```python
from build123d import *

# Parameters (mm, degrees)
F1_DEPTH = 38.1
F2_R     = 88.9
F3_DEPTH = 25.4
F5_DEPTH = 38.1


with BuildPart() as f1:
    # F0 (on Front) → F1 (new body)
    with BuildSketch(Plane.XZ):
        with BuildLine():
            Line((88.9, 0), (0, 0))
            Line((0, 0), (0, -127))
            ThreePointArc((0, -127), (7.4394877579, -144.9605122421), (25.4, -152.4))
            Line((25.4, -152.4), (63.5, -152.4))
            ThreePointArc((63.5, -152.4), (81.4605122421, -144.9605122421), (88.9, -127))
            Line((88.9, -127), (88.9, 0))
        make_face()
    extrude(amount=F1_DEPTH)

    # F2 (on face) → F3 (join)
    with BuildSketch(Plane.XZ.offset(38.1)):
        with Locations((44.45, -114.3)):
            Circle(F2_R)
    extrude(amount=F3_DEPTH)

    # F4 (on face) → F5 (join)
    with BuildSketch(Plane.XZ.offset(63.5)):
        with BuildLine():
            Line((88.9, 0), (0, 0))
            Line((0, 0), (0, -127))
            ThreePointArc((0, -127), (7.4394877579, -144.9605122421), (25.4, -152.4))
            Line((25.4, -152.4), (63.5, -152.4))
            ThreePointArc((63.5, -152.4), (81.4605122421, -144.9605122421), (88.9, -127))
            Line((88.9, -127), (88.9, 0))
        make_face()
    extrude(amount=F5_DEPTH)


solid = f1.part
```
Geometry check sheet. Reference: the model listing, model coordinates, mm. A direction names the side the tool comes from. Coordinates: 2 decimals unless noted, no trailing zeros. Write each loop counter-clockwise with the first axis right and the second up, starting at its lowest first coordinate (ties: lowest second). Pieces come first, ordered by that corner, then holes. Notation, with made-up numbers: M 50,88 L 106,88 A17 cw 106,108 Z; hole C -4.5,75.25 d2. An arc over 180 degrees is marked long. Answer as a JSON object with one key per item and string values.
1. Go/stop test with flat-tipped pins: pin 1 Ø18.5 at (x, z) = (41.5, -10.5) entering from +Y; pin 2 Ø4 at (x, y) = (78, -82.5) entering from -Z; pin 3 Ø12 at (y, z) = (-19, -155) entering from -X; pin 4 Ø12 at (y, z) = (-28.5, -91) entering from +X. Record where each tip stops, or that it passes through.
Answers below:
{"pin 1": "stops at y = 0", "pin 2": "stops at z = -149.11", "pin 3": "stops at x = 12.71", "pin 4": "stops at x = 88.9"}
2. Section check C-C, the plane y = -78. Enter the section's corners in (x, z), plus the area to 3 significant figures.
Answers below:
{"outline": "M 0,-127 A25.4 ccw 25.4,-152.4 L 63.5,-152.4 A25.4 ccw 88.9,-127 L 88.9,0 L 0,0 Z", "area": "13,300 mm²"}
3. Section check D-D, the plane y = -54.5. Enter the section's corners in (x, z).
Answers below:
{"outline": "C 44.45,-114.3 d177.8"}
4. Scan lines: L1, parallel to Y at x = -18.5, z = -94; L2, parallel to Z at x = 54, y = -24.5; L3, parallel to X at y = -28, z = -122. Record each from-to range of solid material in increasing order.
Answers below:
{"L1": "y = -63.5 to -38.1", "L2": "z = -152.4 to 0", "L3": "x = 0 to 88.9"}
5. Section check A-A, the plane z = -114.3. Enter the section's corners in (x, y), plus the area to 3 significant figures.
Answers below:
{"outline": "M -44.45,-63.5 L 0,-63.5 L 0,-101.6 L 88.9,-101.6 L 88.9,-63.5 L 133.35,-63.5 L 133.35,-38.1 L 88.9,-38.1 L 88.9,0 L 0,0 L 0,-38.1 L -44.45,-38.1 Z", "area": "11,300 mm²"}
6. Section check B-B, the plane x = 44.45. Enter the section's corners in (y, z), plus the area to 3 significant figures.
Answers below:
{"outline": "M -101.6,-152.4 L -63.5,-152.4 L -63.5,-203.2 L -38.1,-203.2 L -38.1,-152.4 L 0,-152.4 L 0,0 L -38.1,0 L -38.1,-25.4 L -63.5,-25.4 L -63.5,0 L -101.6,0 Z", "area": "16,100 mm²"}
7. Tool access check on faces 1 (the flat face through (44, -82, -152.4)), 2 (the cylindrical face through (7.24, -82.28, -144.76)), 3 (the flat face through (88.9, -82, -64)), 4 (the flat face through (43, -63.5, -156)). Record the directions out of +Z, -Z, +X, -X, +Y, -Y that give a thin tool (end or side, any length) a straight path to the whole face; none if there is none.
Answers below:
{"face 1": "-Z, +X, -X, -Y", "face 2": "-Z, -X, -Y", "face 3": "+Z, -Z, +X, -Y", "face 4": "-Z, -Y"}
8. Draft check along Y on faces 5 (the flat face through (45, -19, 0)), 6 (the flat face through (44, 0, -75)), 7 (the flat face through (44, -38.1, -14)). Enter one of: released by +Y, released by -Y, zero draft, split by the parting line, or undercut.
Answers below:
{"face 5": "zero draft", "face 6": "released by +Y", "face 7": "undercut"}
